Here's how the part is built. I have some questions about the finished solid (model axes, mm). A direction names the side the tool comes from. Coordinates: 2 decimals unless noted, no trailing zeros. Order: outer loops, then holes, each group sorted by start corner. A loop starts at its lowest first (then second) coordinate and runs counter-clockwise, first axis right, second up. Notation, with made-up numbers: M 65.25,50 L 120.25,50 A22 cw 120.25,58 Z; hole C 18,60 d8. An arc over 180 degrees is marked long. Answer as CSV lines item,"result". Start each with the question number.
```python
from build123d import *

# Parameters (mm, degrees)
SKETCH1_R           = 5.969
BOSS_EXTRUDE1_DEPTH = 1.524
CIRPATTERN1_COUNT   = 3
SKETCH4_R           = 0.381
CUT_EXTRUDE2_DEPTH  = 12.7


with BuildPart() as part:
    # Sketch1 → Boss-Extrude1 (new body)
    with BuildSketch(Plane(origin=(0, 0, 0), x_dir=(1, 0, 0), z_dir=(0, 1, 0))):
        with BuildLine():
            Line((-12.0345, -1.524), (4.697427285, -11.184182722))
            ThreePointArc((4.697427285, -11.184182722), (6.58875, -11.412049758), (7.337072715, -9.660182722))
            Line((7.337072715, -9.660182722), (7.337072715, 9.660182722))
            ThreePointArc((7.337072715, 9.660182722), (6.58875, 11.412049758), (4.697427285, 11.184182722))
            Line((4.697427285, 11.184182722), (-12.0345, 1.524))
            ThreePointArc((-12.0345, 1.524), (-13.1775, 0), (-12.0345, -1.524))
        make_face()
        with Locations(Location((0, 0, 0), (0, 0, 90))):
            Circle(SKETCH1_R, mode=Mode.SUBTRACT)
    extrude(amount=BOSS_EXTRUDE1_DEPTH)

    # Cut-Extrude1 cone 1 section (through the dimple's axis) → Cut-Extrude1 (revolve, cut)
    with BuildSketch(Plane(origin=(-11.65220136, 1.524, 0), x_dir=(0, 0, 1), z_dir=(1, 0, 0))):
        Polygon((0, 0), (1.5875, 0), (0, 1.5875), align=None)
    cut_extrude1 = revolve(axis=Axis((-11.65220136, 1.524, 0), (0, -1, 0)), mode=Mode.SUBTRACT)

    # CirPattern1: Cut-Extrude1 ×3 about axis
    cirpattern1_axis = Axis((0, 0, 0), (0, 1, 0))
    for i in range(1, CIRPATTERN1_COUNT):
        add(cut_extrude1.rotate(cirpattern1_axis, i * 360 / CIRPATTERN1_COUNT), mode=Mode.SUBTRACT)

    # Sketch4 → Cut-Extrude2 (cut)
    with BuildSketch(Plane.XZ):
        with Locations(Location((5.795, -10.03723443, 0), (0, 0, 270))):
            Circle(SKETCH4_R)
        with Locations(Location((-11.59, 0, 0), (0, 0, 270))):
            Circle(SKETCH4_R)
        with Locations(Location((5.795, 10.03723443, 0), (0, 0, 270))):
            Circle(SKETCH4_R)
    extrude(amount=-CUT_EXTRUDE2_DEPTH, mode=Mode.SUBTRACT)


solid = part.part
```
1) Suppose I cut it at B-B on x = 0. Please give me the cut outline in (y, z).
2) If we mould it in two halves opening along Z, with no side actions, what happens to faces 1 (the face through (-13.177, 0.743, -0.029)), 2 (the face through (6.026, 0.458, 10.573)), 3 (the face through (2, 0, 6)), 4 (the face through (-3.551, 0.751, -6.422))? For each: released by +Z, released by -Z, zero draft, split by the parting line, or undercut.
3) I need wall thicknesses on line 1 (X direction, y = 0.2, z = 0); line 2 (X direction, y = 1.1, z = 0); line 3 (X direction, y = 1.2, z = 4.25). Which ranges of each line are inside material? Lowest first, please. Write a range as [from, to].
4) Suppose I cut it at A-A on z = 2.25. Please give me the cut outline in (x, y).
5) Suppose I cut it at D-D on z = -6.75. Please give me the cut outline in (x, y).
6) Which directions (+Z, -Z, +X, -X, +Y, -Y) give clear straight access to the entire face, cutting with the end or side of a thin tool? Please do faces 5 (the face through (6.143, 0.458, -10.505)), 6 (the face through (7.337, 1, 0)).
7) Suppose I cut it at C-C on y = 0.75. Please give me the cut outline in (x, z) (1 decimal), plus the area to 3 significant figures.
Output:
1,outline,"M 0,-8.47 L 1.52,-8.47 L 1.52,-5.97 L 0,-5.97 Z; M 0,5.97 L 1.52,5.97 L 1.52,8.47 L 0,8.47 Z"
2,face 1,"split by the parting line"
2,face 2,"undercut"
2,face 3,"zero draft"
2,face 4,"released by -Z"
3,line 1,"[-13.18, -11.97], [-11.21, -5.97], [5.97, 7.34]"
3,line 2,"[-13.18, -12.82], [-10.49, -5.97], [5.97, 7.34]"
3,line 3,"[-7.31, -4.19], [4.19, 7.34]"
4,outline,"M -10.78,0 L -5.53,0 L -5.53,1.52 L -10.78,1.52 Z; M 5.53,0 L 7.34,0 L 7.34,1.52 L 5.53,1.52 Z"
5,outline,"M -2.98,0 L 7.34,0 L 7.34,1.52 L -2.98,1.52 Z"
6,face 5,"+Y"
6,face 6,"+X, +Y, -Y"
7,outline,"M -12,-1.5 L 4.7,-11.2 A1.6 ccw 7.3,-9.7 L 7.3,9.7 A1.6 ccw 4.7,11.2 L -12,1.5 A1.6 ccw Z; hole C -11.7,0 d1.6; hole C 0,0 d11.9; hole C 5.8,-10.1 d1.6; hole C 5.8,10.1 d1.6"
7,area,"157 mm²"
